from build123d import *

# Parameters (mm, degrees)
BOSS_EXTRUDE2_DEPTH = 20
SKETCH5_W           = 120
SKETCH5_H           = 120
CUT_EXTRUDE1_DEPTH  = 15
FILLET2_R           = 1
FILLET3_R           = 1
FILLET4_R           = 1
FILLET5_R           = 1
CUT_EXTRUDE2_DEPTH  = 5
SKETCH8_W           = 60
SKETCH8_H           = 16
CUT_EXTRUDE5_DEPTH  = 5
SKETCH9_W           = 84
SKETCH9_H           = 40
CUT_EXTRUDE6_DEPTH  = 2.5
SKETCH10_R          = 3
BOSS_EXTRUDE3_DEPTH = 9
CHAMFER1_SIZE       = 2
CUT_EXTRUDE11_DEPTH = 5
CUT_EXTRUDE12_DEPTH = 4
SKETCH17_R          = 3
BOSS_EXTRUDE4_DEPTH = 10.54
SKETCH20_W          = 122.5
SKETCH20_H          = 122.5
CUT_EXTRUDE15_DEPTH = 0.5
FILLET7_R           = 1
FILLET8_R           = 1
FILLET9_R           = 1
FILLET10_R          = 1
SKETCH19_R          = 1.2
CUT_EXTRUDE20_DEPTH = 6
SKETCH18_R          = 1.2
CUT_EXTRUDE21_DEPTH = 6
SKETCH11_R          = 1.025
CUT_EXTRUDE22_DEPTH = 6
SKETCH13_R          = 1.025
CUT_EXTRUDE23_DEPTH = 6
SKETCH12_R          = 1.025
CUT_EXTRUDE24_DEPTH = 6
SKETCH14_R          = 1.025
CUT_EXTRUDE25_DEPTH = 6
SKETCH24_R          = 0.875
CUT_EXTRUDE28_DEPTH = 3
FILLET11_R          = 1
FILLET12_R          = 1


with BuildPart() as part:
    # Sketch4 → Boss-Extrude2 (new body)
    with BuildSketch(Plane(origin=(0, 0, 0), x_dir=(1, 0, 0), z_dir=(0, 1, 0))):
        with BuildLine():
            Line((-59.5, 65), (59.5, 65))
            ThreePointArc((59.5, 65), (63.389087297, 63.389087297), (65, 59.5))
            Line((65, 59.5), (65, -59.5))
            ThreePointArc((65, -59.5), (63.389087297, -63.389087297), (59.5, -65))
            Line((59.5, -65), (-59.5, -65))
            ThreePointArc((-59.5, -65), (-63.389087297, -63.389087297), (-65, -59.5))
            Line((-65, -59.5), (-65, 59.5))
            ThreePointArc((-65, 59.5), (-63.389087297, 63.389087297), (-59.5, 65))
        make_face()
    extrude(amount=BOSS_EXTRUDE2_DEPTH)

    # Sketch5 → Cut-Extrude1 (cut)
    with BuildSketch(Plane(origin=(0, 20, 0), x_dir=(1, 0, 0), z_dir=(0, 1, 0))):
        Rectangle(SKETCH5_W, SKETCH5_H)
    extrude(amount=-CUT_EXTRUDE1_DEPTH, mode=Mode.SUBTRACT)

    # Fillet2
    fillet2_edges = [part.edges().sort_by_distance(p)[0] for p in [
        (-60, 12.5, -60),
    ]]
    fillet(fillet2_edges, radius=FILLET2_R)

    # Fillet3
    fillet3_edges = [part.edges().sort_by_distance(p)[0] for p in [
        (60, 12.5, -60),
    ]]
    fillet(fillet3_edges, radius=FILLET3_R)

    # Fillet4
    fillet4_edges = [part.edges().sort_by_distance(p)[0] for p in [
        (-60, 12.5, 60),
    ]]
    fillet(fillet4_edges, radius=FILLET4_R)

    # Fillet5
    fillet5_edges = [part.edges().sort_by_distance(p)[0] for p in [
        (60, 12.5, 60),
    ]]
    fillet(fillet5_edges, radius=FILLET5_R)

    # Sketch6 → Cut-Extrude2 (cut)
    with BuildSketch(Plane(origin=(0, 5, 0), x_dir=(1, 0, 0), z_dir=(0, 1, 0))):
        with BuildLine():
            Line((-19, 10), (19, 10.074775785))
            ThreePointArc((19, 10.074775785), (22.00520382, 8.829979605), (23.25, 5.824775785))
            Line((23.25, 5.824775785), (23.25, -43.25))
            ThreePointArc((23.25, -43.25), (22.00520382, -46.25520382), (19, -47.5))
            Line((19, -47.5), (-19, -47.5))
            ThreePointArc((-19, -47.5), (-22.00520382, -46.25520382), (-23.25, -43.25))
            Line((-23.25, -43.25), (-23.25, 5.75))
            ThreePointArc((-23.25, 5.75), (-22.00520382, 8.75520382), (-19, 10))
        make_face()
    extrude(amount=-CUT_EXTRUDE2_DEPTH, mode=Mode.SUBTRACT)

    # Sketch8 → Cut-Extrude5 (cut)
    with BuildSketch(Plane(origin=(0, 5, 0), x_dir=(1, 0, 0), z_dir=(0, 1, 0))):
        with Locations((0, 38)):
            Rectangle(SKETCH8_W, SKETCH8_H)
    extrude(amount=-CUT_EXTRUDE5_DEPTH, mode=Mode.SUBTRACT)

    # Sketch9 → Cut-Extrude6 (cut)
    with BuildSketch(Plane(origin=(0, 5, 0), x_dir=(1, 0, 0), z_dir=(0, 1, 0))):
        with Locations((0, 38)):
            Rectangle(SKETCH9_W, SKETCH9_H)
    extrude(amount=-CUT_EXTRUDE6_DEPTH, mode=Mode.SUBTRACT)

    # Sketch10 → Boss-Extrude3 (add)
    with BuildSketch(Plane(origin=(0, 2.5, 0), x_dir=(1, 0, 0), z_dir=(0, 1, 0))):
        with Locations((37.5, 53.5)):
            Circle(SKETCH10_R)
        with Locations((-37.5, 53.5)):
            Circle(SKETCH10_R)
        with Locations((-37.5, 22.5)):
            Circle(SKETCH10_R)
        with Locations((37.5, 22.5)):
            Circle(SKETCH10_R)
    extrude(amount=BOSS_EXTRUDE3_DEPTH)

    # Chamfer1
    chamfer1_edges = [part.edges().sort_by_distance(p)[0] for p in [
        (30, 0, -38),
        (0, 0, -30),
        (-30, 0, -38),
        (0, 0, -46),
    ]]
    chamfer(chamfer1_edges, length=CHAMFER1_SIZE)

    # Sketch15 → Cut-Extrude11 (cut)
    with BuildSketch(Plane(origin=(0, 0, -65), x_dir=(-1, 0, 0), z_dir=(0, 0, -1))):
        with BuildLine():
            Line((-45.118313756, 20), (-48.381686244, 20))
            ThreePointArc((-48.381686244, 20), (-46.75, 17.44), (-45.118313756, 20))
        make_face()
    extrude(amount=-CUT_EXTRUDE11_DEPTH, mode=Mode.SUBTRACT)

    # Sketch16 → Cut-Extrude12 (cut)
    with BuildSketch(Plane(origin=(0, 0, -65), x_dir=(-1, 0, 0), z_dir=(0, 0, -1))):
        with BuildLine():
            Line((-43.847862856, 20), (-49.652137144, 20))
            ThreePointArc((-49.652137144, 20), (-46.75, 16.24), (-43.847862856, 20))
        make_face()
    extrude(amount=-CUT_EXTRUDE12_DEPTH, mode=Mode.SUBTRACT)

    # Sketch17 → Boss-Extrude4 (add)
    with BuildSketch(Plane(origin=(0, 5, 0), x_dir=(1, 0, 0), z_dir=(0, 1, 0))):
        with Locations((49.7, -15.8)):
            Circle(SKETCH17_R)
        with Locations((-49.8, -15.8)):
            Circle(SKETCH17_R)
    extrude(amount=BOSS_EXTRUDE4_DEPTH)

    # Sketch20 → Cut-Extrude15 (cut)
    with BuildSketch(Plane(origin=(0, 20, 0), x_dir=(1, 0, 0), z_dir=(0, 1, 0))):
        with BuildLine():
            Line((-59.5, -65), (59.5, -65))
            ThreePointArc((59.5, -65), (63.389087297, -63.389087297), (65, -59.5))
            Line((65, -59.5), (65, 59.5))
            ThreePointArc((65, 59.5), (63.389087297, 63.389087297), (59.5, 65))
            Line((59.5, 65), (-59.5, 65))
            ThreePointArc((-59.5, 65), (-63.389087297, 63.389087297), (-65, 59.5))
            Line((-65, 59.5), (-65, -59.5))
            ThreePointArc((-65, -59.5), (-63.389087297, -63.389087297), (-59.5, -65))
        make_face()
        Rectangle(SKETCH20_W, SKETCH20_H, mode=Mode.SUBTRACT)
    extrude(amount=-CUT_EXTRUDE15_DEPTH, mode=Mode.SUBTRACT)

    # Fillet7
    fillet7_edges = [part.edges().sort_by_distance(p)[0] for p in [
        (61.25, 19.75, 61.25),
    ]]
    fillet(fillet7_edges, radius=FILLET7_R)

    # Fillet8
    fillet8_edges = [part.edges().sort_by_distance(p)[0] for p in [
        (-61.25, 19.75, 61.25),
    ]]
    fillet(fillet8_edges, radius=FILLET8_R)

    # Fillet9
    fillet9_edges = [part.edges().sort_by_distance(p)[0] for p in [
        (-61.25, 19.75, -61.25),
    ]]
    fillet(fillet9_edges, radius=FILLET9_R)

    # Fillet10
    fillet10_edges = [part.edges().sort_by_distance(p)[0] for p in [
        (61.25, 19.75, -61.25),
    ]]
    fillet(fillet10_edges, radius=FILLET10_R)

    # Sketch19 → Cut-Extrude20 (cut)
    with BuildSketch(Plane(origin=(0, 15.54, 0), x_dir=(1, 0, 0), z_dir=(0, 1, 0))):
        with Locations((49.7, -15.8)):
            Circle(SKETCH19_R)
    extrude(amount=-CUT_EXTRUDE20_DEPTH, mode=Mode.SUBTRACT)

    # Sketch18 → Cut-Extrude21 (cut)
    with BuildSketch(Plane(origin=(0, 15.54, 0), x_dir=(1, 0, 0), z_dir=(0, 1, 0))):
        with Locations((-49.8, -15.8)):
            Circle(SKETCH18_R)
    extrude(amount=-CUT_EXTRUDE21_DEPTH, mode=Mode.SUBTRACT)

    # Sketch11 → Cut-Extrude22 (cut)
    with BuildSketch(Plane(origin=(0, 11.5, 0), x_dir=(1, 0, 0), z_dir=(0, 1, 0))):
        with Locations((-37.5, 53.5)):
            Circle(SKETCH11_R)
    extrude(amount=-CUT_EXTRUDE22_DEPTH, mode=Mode.SUBTRACT)

    # Sketch13 → Cut-Extrude23 (cut)
    with BuildSketch(Plane(origin=(0, 11.5, 0), x_dir=(1, 0, 0), z_dir=(0, 1, 0))):
        with Locations((37.5, 53.5)):
            Circle(SKETCH13_R)
    extrude(amount=-CUT_EXTRUDE23_DEPTH, mode=Mode.SUBTRACT)

    # Sketch12 → Cut-Extrude24 (cut)
    with BuildSketch(Plane(origin=(0, 11.5, 0), x_dir=(1, 0, 0), z_dir=(0, 1, 0))):
        with Locations((-37.5, 22.5)):
            Circle(SKETCH12_R)
    extrude(amount=-CUT_EXTRUDE24_DEPTH, mode=Mode.SUBTRACT)

    # Sketch14 → Cut-Extrude25 (cut)
    with BuildSketch(Plane(origin=(0, 11.5, 0), x_dir=(1, 0, 0), z_dir=(0, 1, 0))):
        with Locations((37.5, 22.5)):
            Circle(SKETCH14_R)
    extrude(amount=-CUT_EXTRUDE25_DEPTH, mode=Mode.SUBTRACT)

    # Sketch24 → Cut-Extrude28 (cut)
    with BuildSketch(Plane(origin=(0, 5, 0), x_dir=(1, 0, 0), z_dir=(0, 1, 0))):
        with Locations((23, 10.768693946)):
            Circle(SKETCH24_R)
        with Locations((-23, 10.768693946)):
            Circle(SKETCH24_R)
        with Locations((-23, -48.231306054)):
            Circle(SKETCH24_R)
        with Locations((23, -48.231306054)):
            Circle(SKETCH24_R)
    extrude(amount=-CUT_EXTRUDE28_DEPTH, mode=Mode.SUBTRACT)

    # Fillet11
    fillet11_edges = [part.edges().sort_by_distance(p)[0] for p in [
        (-52.8, 5, 15.8),
    ]]
    fillet(fillet11_edges, radius=FILLET11_R)

    # Fillet12
    fillet12_edges = [part.edges().sort_by_distance(p)[0] for p in [
        (46.7, 5, 15.8),
    ]]
    fillet(fillet12_edges, radius=FILLET12_R)


solid = part.part
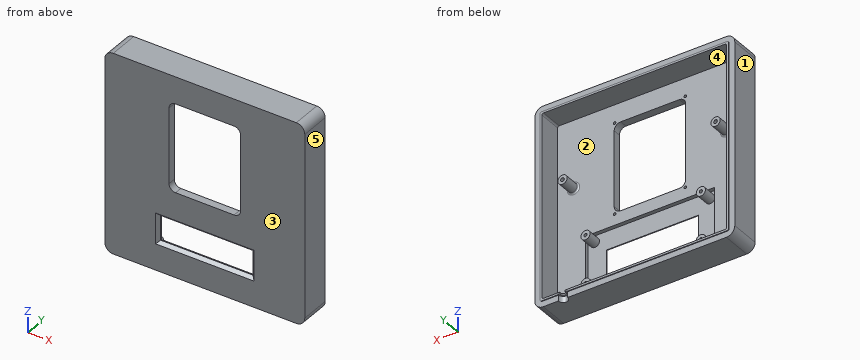
Can you work these out from the model? Positions are in its coordinate system, mm. Face numbers are marked on the shaded views. A direction names the side the tool comes from. Give positions to 0.01 mm unless a question says otherwise; leave off trailing zeros. Loops run counter-clockwise (first coordinate to the right, second up) from the corner with the lowest first, then second, coordinate; pieces in that order, holes last. Notation, with made-up numbers: M -12.75,-17.75 L 36.25,-17.75 A17 ccw 36.25,2.25 Z; hole C 89,78.5 d4. An arc over 180 degrees is marked long. One line per item, written item: value. Start each with the question number.
1) If we section it at A-A, the plane x = -15: Write out the boundary of the cut face in (y, z), and give its area (3 significant figures).
2) Thinking about a two-plate mould opening in X: for the marked faces 1, 2 and 3, which applies, +X half, -X half, draft (parallel to the pull), parting line (faces both ways), or undercut?
3) On a 3-axis mill with a long thin cutter (end or side, diameter ignored), from which of +Z, -Z, +X, -X, +Y, -Y can I reach the whole of each face in a straight line? I mean the marked faces 4 and 5. Say none if no direction works.
4) I'm going to push flat-ended pins straight in: pin 1 (6.5 mm diameter, centred on x = 36, z = -54.5, fed in from +Y); pin 2 (3 mm diameter, centred on x = 46, y = 19, fed in from -Z); pin 3 (1.4 mm diameter, centred on x = -23, z = 48, fed in from +Y). Where does each tip first touch, or does it pass through?
5) If we section it at B-B, the plane x = -2: Write out the boundary of the cut face in (y, z), and give its area (3 significant figures).
6) If I drill on line 1 (X direction, y = 10.1, z = -53.5) (3 decimals); line 2 (Z direction, x = -49.8, y = 13.6); line 3 (Z direction, x = -29.5, y = 15), over which ranges is the centre line in solid material (lowest first)? Write a range as [from, to].
Completed:
1. outline: M 0,-65 L 19.5,-65 L 19.5,-61.25 L 20,-61.25 L 20,-60 L 5,-60 L 5,-58 L 2.5,-58 L 2.5,-46 L 2,-46 L 0,-48 Z; M 0,-28 L 2,-30 L 2.5,-30 L 2.5,-18 L 5,-18 L 5,-10.01 L 0,-10.01 Z; M 0,47.5 L 5,47.5 L 5,60 L 20,60 L 20,61.25 L 19.5,61.25 L 19.5,65 L 0,65 Z
1. area: 365 mm^2
2. face 1: -X half
2. face 2: undercut
2. face 3: draft
3. face 4: +Y
3. face 5: +Z, -Z, +X, +Y, -Y
4. pin 1: stops at y = 11.5
4. pin 2: stops at z = -61
4. pin 3: stops at y = 5
5. outline: M 0,-65 L 19.5,-65 L 19.5,-61.25 L 20,-61.25 L 20,-60 L 5,-60 L 5,-58 L 2.5,-58 L 2.5,-46 L 2,-46 L 0,-48 Z; M 0,-28 L 2,-30 L 2.5,-30 L 2.5,-18 L 5,-18 L 5,-10.03 L 0,-10.03 Z; M 0,47.5 L 5,47.5 L 5,60 L 20,60 L 20,61.25 L 19.5,61.25 L 19.5,65 L 0,65 Z
5. area: 365 mm^2
6. line 1: x = [-65, -60], [-40.5, -38.525], [-36.475, -34.5], [34.5, 36.475], [38.525, 40.5], [60, 65]
6. line 2: z = [-65, -60], [12.8, 14.6], [17, 18.8], [60, 65]
6. line 3: z = [-65, -60], [60, 65]
